Design review of the part built by this model. Coordinates are the model's own, in mm. Give positions to 0.01 mm unless a question says otherwise; leave off trailing zeros. Loops run counter-clockwise (first coordinate to the right, second up) from the corner with the lowest first, then second, coordinate; pieces in that order, holes last. Notation, with made-up numbers: (-19.5, -35) -> (1.5, -35) arc R35 cw to (1.5, -3) -> close; hole circle Ø1 at (46.25, 22.25). An arc over 180 degrees is marked (long way). Use a Markdown table: item, result. Add a question column.
1. For pin 1 Ø1 at (x, z) = (13, 12) entering from -Y (3 decimals), flat-tipped, find the tip position at first contact; note if it passes through.
2. Add section B-B (y = 0). State the section outline as (x, z) points, and give its area (3 significant figures).
3. Add section A-A (x = 12.8). State the section outline as (y, z) points.
4. Add section C-C (z = 12). State the section outline as (x, y) points, and give its area (3 significant figures).
5. To check wall thickness, follow line 1 (Z direction, x = 13.8, y = -1); line 2 (Y direction, x = 13.25, z = 12.5); line 3 (Z direction, x = 13.6, y = -1.05). State the ranges of each line that lie inside material, in increasing order.
```python
from build123d import *

# Parameters (mm, degrees)
F0_W        = 2.54
F0_H        = 2.3375834556
F1_DEPTH    = 25.4
F2_T1_DEPTH = 67.8607478943
F3_R        = 5.08
F4_T1_DEPTH = 20.8515396399


# Not quite as in the source:
# - a fillet or chamfer that OpenCascade refuses, or shapes differently, is made with other operations: its cross-section is extruded or revolved along the edge and cut away or added


with BuildPart() as f1:
    # F0 (on Top) → F1 (new body)
    with BuildSketch(Plane.XY):
        with Locations((13.1794903427, -0.4677381366)):
            Rectangle(F0_W, F0_H)
    extrude(amount=F1_DEPTH)

    # F2: chamfer of 12.7 on 1 edges, made by hand

    # F2_s2 → F2_t1 (cut)
    with BuildSketch(Plane.YZ.offset(-20.7508836044)):
        Polygon((0.7010535912, 12.7), (-11.9989464088, 25.4), (0.7010535912, 25.4), align=None)
    extrude(amount=F2_T1_DEPTH, mode=Mode.SUBTRACT)

    # F3
    f3_edges = [f1.edges().sort_by_distance(p)[0] for p in [
        (13.17949, 0.701054, 12.7),
    ]]
    fillet(f3_edges, radius=F3_R)

    # F4: fillet of radius 5.08 on 1 edges, made by hand

    # F4_s2 → F4_t1 (cut)
    with BuildSketch(Plane.YZ.offset(2.7537205228)):
        with BuildLine():
            ThreePointArc((-0.7868439604, 14.1878975516), (-1.4194711353, 12.8443576208), (-1.6365298645, 11.3752755277))
            Line((-1.6365298645, 11.3752755277), (-1.6365298645, 15.0375834557))
            Line((-1.6365298645, 15.0375834557), (-0.7868439604, 14.1878975516))
        make_face()
    extrude(amount=F4_T1_DEPTH, mode=Mode.SUBTRACT)


solid = f1.part
```
Taken from the geometry:
| question | item | result |
|---|---|---|
| 1 | pin 1 | stops at y = -1.635 |
| 2 | outline | (11.91, 0) -> (14.45, 0) -> (14.45, 13.17) -> (11.91, 13.17) -> close |
| 2 | area | 33.5 mm^2 |
| 3 | outline | (-1.64, 0) -> (0.7, 0) -> (0.7, 10.6) arc R5.08 ccw to (-0.79, 14.19) arc R5.08 ccw to (-1.64, 11.38) -> close |
| 4 | outline | (11.91, -1.6) -> (14.45, -1.6) -> (14.45, 0.5) -> (11.91, 0.5) -> close |
| 4 | area | 5.34 mm^2 |
| 5 | line 1 | z = 0 to 13.84 |
| 5 | line 2 | y = -1.51 to 0.33 |
| 5 | line 3 | z = 0 to 13.74 |
